Input: part model. Units: mm. Frame: model coordinates. Coordinates: 2 decimals unless noted, no trailing zeros. Loops run counter-clockwise (first coordinate to the right, second up) from the corner with the lowest first, then second, coordinate; pieces in that order, holes last. Notation, with made-up numbers: M 12,24.5 L 23,24.5 A20 ccw 23,31.5 Z; hole C 16,9 d7. An arc over 180 degrees is marked long. Use a Markdown table: item, result. Add a question column.
1. Draft query along Y for faces 1 (the flat face through (-12, 1, 3)), 2 (the cylindrical face through (-50.95, -47.99, 1.52)), 3 (the cylindrical face through (-15.923, -12.278, 1.479)). Return one class per face: +Y half, -Y half, draft (parallel to the pull), parting line (faces both ways), or undercut.
2. Section C-C on x = -15.5. Output: boundary loops of the cut face in (y, z).
3. Section D-D on y = -15.5. Output: boundary loops of the cut face in (x, z), then the cut area to 3 significant figures.
4. Line query: L1, parallel to Y at x = 15.5, z = 2.2; L2, parallel to Y at x = -41.3, z = 1.2; L3, parallel to X at y = 39.5, z = 1.3. Output: solid intervals per line, ascending. Write a range as [from, to].
5. Pin query (flat end, axial travel): pin 1 (5 mm diameter, centred on x = -41.3, y = -38.5, fed in from -Z). Return the tip coordinate at first contact, or that it passes through.
6. Section A-A on y = 0. Output: boundary loops of the cut face in (x, z).
7. Section B-B on z = 2. State how many separate pieces and enclosed holes the cut face has, then the cut area to 3 significant figures.
```python
from build123d import *

# Parameters (mm, degrees)
CROQUIS1_W              = 85
CROQUIS1_H              = 102
CROQUIS1_R              = 4.5
CROQUIS1_R_2            = 3.25
CROQUIS1_R_3            = 3.15
SALIENTE_EXTRUIR1_DEPTH = 3
REDONDEO1_R             = 10


with BuildPart() as part:
    # Croquis1 → Saliente-Extruir1 (new body)
    with BuildSketch(Plane.XY):
        with Locations((-11.3, 0)):
            Rectangle(CROQUIS1_W, CROQUIS1_H)
        Circle(CROQUIS1_R, mode=Mode.SUBTRACT)
        with Locations((15.5, 15.5)):
            Circle(CROQUIS1_R_2, mode=Mode.SUBTRACT)
        with Locations(Location((-15.5, 15.5, 0), (0, 0, 180))):
            Circle(CROQUIS1_R_2, mode=Mode.SUBTRACT)
        with Locations(Location((15.5, -15.5, 0), (0, 0, 180))):
            Circle(CROQUIS1_R_2, mode=Mode.SUBTRACT)
        with Locations((-15.5, -15.5)):
            Circle(CROQUIS1_R_2, mode=Mode.SUBTRACT)
        with Locations((-41.3, 38.5)):
            Circle(CROQUIS1_R_3, mode=Mode.SUBTRACT)
        with Locations((18.7, 38.5)):
            Circle(CROQUIS1_R_3, mode=Mode.SUBTRACT)
        with Locations(Location((18.7, -38.5, 0), (0, 0, 180))):
            Circle(CROQUIS1_R_3, mode=Mode.SUBTRACT)
        with Locations(Location((-41.3, -38.5, 0), (0, 0, 180))):
            Circle(CROQUIS1_R_3, mode=Mode.SUBTRACT)
    extrude(amount=SALIENTE_EXTRUIR1_DEPTH)

    # Redondeo1
    redondeo1_edges = [part.edges().sort_by_distance(p)[0] for p in [
        (-53.8, 51, 1.5),
        (31.2, 51, 1.5),
        (31.2, -51, 1.5),
        (-53.8, -51, 1.5),
    ]]
    fillet(redondeo1_edges, radius=REDONDEO1_R)


solid = part.part
```
Answers below:
| question | item | result |
|---|---|---|
| 1 | face 1 | draft |
| 1 | face 2 | -Y half |
| 1 | face 3 | undercut |
| 2 | outline | M -51,0 L -18.75,0 L -18.75,3 L -51,3 Z; M -12.25,0 L 12.25,0 L 12.25,3 L -12.25,3 Z; M 18.75,0 L 51,0 L 51,3 L 18.75,3 Z |
| 3 | outline | M -53.8,0 L -18.75,0 L -18.75,3 L -53.8,3 Z; M -12.25,0 L 12.25,0 L 12.25,3 L -12.25,3 Z; M 18.75,0 L 31.2,0 L 31.2,3 L 18.75,3 Z |
| 3 | area | 216 mm² |
| 4 | L1 | y = [-51, -18.75], [-12.25, 12.25], [18.75, 51] |
| 4 | L2 | y = [-51, -41.65], [-35.35, 35.35], [41.65, 51] |
| 4 | L3 | x = [-53.8, -44.29], [-38.31, 15.71], [21.69, 31.2] |
| 5 | pin 1 | passes through |
| 6 | outline | M -53.8,0 L -4.5,0 L -4.5,3 L -53.8,3 Z; M 4.5,0 L 31.2,0 L 31.2,3 L 4.5,3 Z |
| 7 | separate pieces | 1 |
| 7 | enclosed holes | 9 |
| 7 | area | 8,260 mm² |
